Read the model definition and answer for the solid it produces. Units are mm, in the model's axes. A direction names the side the tool comes from. Coordinates: 2 decimals unless noted, no trailing zeros. Write each loop counter-clockwise with the first axis right and the second up, starting at its lowest first coordinate (ties: lowest second). Pieces come first, ordered by that corner, then holes. Notation, with made-up numbers: (-1, 5) -> (51, 5) arc R36 cw to (51, 39) -> close; hole circle Ø5 at (59.5, 72). An arc over 180 degrees is marked (long way). Answer as a JSON object with one key per item and string values. Group by question number.
(1) For a pull along X with two mould halves and no side action, classify faces 4 (the face through (-20.892, 1, 5)), 5 (the face through (-20, 1, 0)), 6 (the face through (-19.09, 1.15, 8.03)) as +X half, -X half, draft (parallel to the pull), parting line (faces both ways), or undercut.
(2) Find section B-B (y = 1.75). Give the vertices of the cut face in (x, z).
(3) Find section C-C (x = -17.75). Give the vertices of the cut face in (y, z), then the cut area to 3 significant figures.
(4) Find section D-D (z = 8.5). Give the vertices of the cut face in (x, y), then the cut area to 3 significant figures.
(5) Find section A-A (z = 3). Give the vertices of the cut face in (x, y).
(6) Which of the six approach directions +Z, -Z, +X, -X, +Y, -Y give full straight-line access (tool end or side, diameter ignored) to faces 1 (the face through (-18, 2.681, 2)), 2 (the face through (-14.292, 1, 5)), 3 (the face through (-18, 1, 6))?
(7) A flat-ended cylindrical pin translates along its axis: P1, Ø2.5, axis at x = -17.59, y = 1.08, coming from the -Z side. Find the tip coordinate at first contact, or state that the pin passes through.
(8) Straight lines are drawn through the part: L1, parallel to Y at x = -16.5, z = 1.25; L2, parallel to X at y = 1, z = 6.75; L3, parallel to X at y = 0.25, z = 3.25. For each, find the intervals that lie inside material, in ascending order.
from build123d import *

# Parameters (mm, degrees)
CROQUIS1_W              = 6.6
CROQUIS1_H              = 6.6
SALIENTE_EXTRUIR1_DEPTH = 10
CROQUIS2_R              = 1.5
CORTAR_EXTRUIR1_DEPTH   = 4
CROQUIS3_W              = 3.2
CROQUIS3_H              = 3.2
CORTAR_EXTRUIR2_DEPTH   = 4


with BuildPart() as part:
    # Croquis1 → Saliente-Extruir1 (new body)
    with BuildSketch(Plane.XY):
        with Locations((-17.592123702, 1.080530973)):
            Rectangle(CROQUIS1_W, CROQUIS1_H)
    extrude(amount=SALIENTE_EXTRUIR1_DEPTH)

    # Croquis2 → Cortar-Extruir1 (cut)
    with BuildSketch(Plane.XY.offset(10)):
        with Locations((-17.592123702, 1.080530973)):
            Circle(CROQUIS2_R)
    extrude(amount=-CORTAR_EXTRUIR1_DEPTH, mode=Mode.SUBTRACT)

    # Croquis3 → Cortar-Extruir2 (cut)
    with BuildSketch(Plane(origin=(0, 0, 0), x_dir=(-1, 0, 0), z_dir=(0, 0, -1))):
        with Locations((17.592123702, 1.080530973)):
            Rectangle(CROQUIS3_W, CROQUIS3_H)
    extrude(amount=-CORTAR_EXTRUIR2_DEPTH, mode=Mode.SUBTRACT)


solid = part.part
Results below:
{
 "1": {"face 4": "-X half", "face 5": "draft", "face 6": "undercut"},
 "2": {"outline": "(-20.89, 0) -> (-19.19, 0) -> (-19.19, 4) -> (-15.99, 4) -> (-15.99, 0) -> (-14.29, 0) -> (-14.29, 10) -> (-16.25, 10) -> (-16.25, 6) -> (-18.93, 6) -> (-18.93, 10) -> (-20.89, 10) -> close"},
 "3": {"outline": "(-2.22, 0) -> (-0.52, 0) -> (-0.52, 4) -> (2.68, 4) -> (2.68, 0) -> (4.38, 0) -> (4.38, 10) -> (2.57, 10) -> (2.57, 6) -> (-0.41, 6) -> (-0.41, 10) -> (-2.22, 10) -> close", "area": "41.3 mm2"},
 "4": {"outline": "(-20.89, -2.22) -> (-14.29, -2.22) -> (-14.29, 4.38) -> (-20.89, 4.38) -> close; hole circle Ø3 at (-17.59, 1.08)", "area": "36.5 mm2"},
 "5": {"outline": "(-20.89, -2.22) -> (-14.29, -2.22) -> (-14.29, 4.38) -> (-20.89, 4.38) -> close; hole (-19.19, -0.52) -> (-15.99, -0.52) -> (-15.99, 2.68) -> (-19.19, 2.68) -> close"},
 "6": {"face 1": "-Z", "face 2": "+Z, -Z, +X, +Y, -Y", "face 3": "+Z"},
 "7": {"P1": "stops at z = 4"},
 "8": {"L1": "y = -2.22 to -0.52, 2.68 to 4.38", "L2": "x = -20.89 to -19.09, -16.09 to -14.29", "L3": "x = -20.89 to -19.19, -15.99 to -14.29"}
}
